Source: CAD feature listing. Evaluate the final solid. Frame: model axes, mm. A direction names the side the tool comes from. Round coordinates to 2 decimals unless told otherwise and drop trailing zeros. Order: outer loops, then holes, each group sorted by start corner. A loop starts at its lowest first (then second) coordinate and runs counter-clockwise, first axis right, second up. Notation, with made-up numbers: (65, -18) -> (122, -18) arc R34 cw to (122, 13) -> close; hole circle Ø10 at (18.25, 51). An arc over 180 degrees is marked (long way). Use a Markdown table: item, result. Add a question column.
```python
from build123d import *

# Parameters (mm, degrees)
BOSS_EXTRUDE1_DEPTH = 5


with BuildPart() as part:
    # Sketch1 → Boss-Extrude1 (new body)
    with BuildSketch(Plane.XY):
        with BuildLine():
            Line((105.70441989, 0), (143.20441989, 0))
            ThreePointArc((143.20441989, 0), (150.275487701, 2.928932188), (153.20441989, 10))
            Line((153.20441989, 10), (153.20441989, 15))
            ThreePointArc((153.20441989, 15), (150.275487701, 22.071067812), (143.20441989, 25))
            Line((143.20441989, 25), (-41.79558011, 25))
            ThreePointArc((-41.79558011, 25), (-48.866647922, 22.071067812), (-51.79558011, 15))
            Line((-51.79558011, 15), (-51.79558011, 10))
            ThreePointArc((-51.79558011, 10), (-48.866647922, 2.928932188), (-41.79558011, 0))
            Line((-41.79558011, 0), (-4.29558011, 0))
            ThreePointArc((-4.29558011, 0), (-0.760046205, -1.464466094), (0.70441989, -5))
            Line((0.70441989, -5), (0.70441989, -95))
            ThreePointArc((0.70441989, -95), (2.168885984, -98.535533906), (5.70441989, -100))
            Line((5.70441989, -100), (95.70441989, -100))
            ThreePointArc((95.70441989, -100), (99.239953795, -98.535533906), (100.70441989, -95))
            Line((100.70441989, -95), (100.70441989, -5))
            ThreePointArc((100.70441989, -5), (102.168885984, -1.464466094), (105.70441989, 0))
        make_face()
        with BuildLine():
            Line((-41.79558011, 20), (143.20441989, 20))
            ThreePointArc((143.20441989, 20), (146.739953795, 18.535533906), (148.20441989, 15))
            Line((148.20441989, 15), (148.20441989, 10))
            ThreePointArc((148.20441989, 10), (146.739953795, 6.464466094), (143.20441989, 5))
            Line((143.20441989, 5), (-41.79558011, 5))
            ThreePointArc((-41.79558011, 5), (-45.331114016, 6.464466094), (-46.79558011, 10))
            Line((-46.79558011, 10), (-46.79558011, 15))
            ThreePointArc((-46.79558011, 15), (-45.331114016, 18.535533906), (-41.79558011, 20))
        make_face(mode=Mode.SUBTRACT)
    extrude(amount=BOSS_EXTRUDE1_DEPTH)


solid = part.part
```
1) Section D-D on y = -22.5. Output: boundary loops of the cut face in (x, z).
2) Section C-C on y = 17.5. Output: boundary loops of the cut face in (x, z), then the cut area to 3 significant figures.
3) First-contact query: pin 1 Ø1 at (y, z) = (-49, 4.5) entering from -X; pin 2 Ø1.5 at (x, y) = (6.5, -67) entering from -Z; pin 3 Ø2.5 at (y, z) = (-56.5, 1.5) entering from +X; pin 4 Ø1.5 at (y, z) = (-2.5, 3.5) entering from +X. Flat tips, straight axial feed; report the tip coordinate or a pass-through.
4) Line query: probe 1 along Y at (x, z) = (31, 2.1); probe 2 along Y at (x, z) = (113, 2.8); probe 3 along X at (y, z) = (-81.5, 1.4). Output: solid intervals per line, ascending. Write a range as from..to.
5) Reachability of faces 1 (the cylindrical face through (146.701, 18.574, 2.465)), 2 (the flat face through (100.704, -51, 2)), 3 (the flat face through (-51.796, 13, 2)), 4 (the flat face through (-23, 0, 2)) from +Z, -Z, +X, -X, +Y, -Y: full face, straight path, thin tool, end or side. Return the list, or none.
6) Section B-B on z = 1.45. Output: boundary loops of the cut face in (x, y), then the cut area to 3 significant figures.
7) Draft query along Y for faces 5 (the flat face through (49, -51, 5)), 6 (the flat face through (50, -100, 2)), 7 (the cylindrical face through (146.779, 6.504, 2.465)), 8 (the flat face through (52, 25, 2)). Return one class per face: pulls with the +Y half, pulls with the -Y half, needs draft (parallel to the pull), parting line crosses it, or undercut.
8) Section A-A on x = 90. Output: boundary loops of the cut face in (y, z).
Conclusion:
| question | item | result |
|---|---|---|
| 1 | outline | (0.7, 0) -> (100.7, 0) -> (100.7, 5) -> (0.7, 5) -> close |
| 2 | outline | (-51.48, 0) -> (-46.13, 0) -> (-46.13, 5) -> (-51.48, 5) -> close; (147.53, 0) -> (152.89, 0) -> (152.89, 5) -> (147.53, 5) -> close |
| 2 | area | 53.5 mm^2 |
| 3 | pin 1 | stops at x = 0.7 |
| 3 | pin 2 | stops at z = 0 |
| 3 | pin 3 | stops at x = 100.7 |
| 3 | pin 4 | stops at x = 101.9 |
| 4 | probe 1 | y = -100..5, 20..25 |
| 4 | probe 2 | y = 0..5, 20..25 |
| 4 | probe 3 | x = 0.7..100.7 |
| 5 | face 1 | +Z, -Z |
| 5 | face 2 | +Z, -Z, +X, -Y |
| 5 | face 3 | +Z, -Z, -X, +Y, -Y |
| 5 | face 4 | +Z, -Z, -X, -Y |
| 6 | outline | (-51.8, 10) arc R10 ccw to (-41.8, 0) -> (-4.3, 0) arc R5 cw to (0.7, -5) -> (0.7, -95) arc R5 ccw to (5.7, -100) -> (95.7, -100) arc R5 ccw to (100.7, -95) -> (100.7, -5) arc R5 cw to (105.7, 0) -> (143.2, 0) arc R10 ccw to (153.2, 10) -> (153.2, 15) arc R10 ccw to (143.2, 25) -> (-41.8, 25) arc R10 ccw to (-51.8, 15) -> close; hole (-46.8, 10) arc R5 ccw to (-41.8, 5) -> (143.2, 5) arc R5 ccw to (148.2, 10) -> (148.2, 15) arc R5 ccw to (143.2, 20) -> (-41.8, 20) arc R5 ccw to (-46.8, 15) -> close |
| 6 | area | 12,100 mm^2 |
| 7 | face 5 | needs draft |
| 7 | face 6 | pulls with the -Y half |
| 7 | face 7 | undercut |
| 7 | face 8 | pulls with the +Y half |
| 8 | outline | (-100, 0) -> (5, 0) -> (5, 5) -> (-100, 5) -> close; (20, 0) -> (25, 0) -> (25, 5) -> (20, 5) -> close |
